Work out the finished part from the listing and answer in its coordinate system (mm). A direction names the side the tool comes from. Coordinates: 2 decimals unless noted, no trailing zeros. Write each loop counter-clockwise with the first axis right and the second up, starting at its lowest first coordinate (ties: lowest second). Pieces come first, ordered by that corner, then holes. Notation, with made-up numbers: (86.25, 8) - (110.25, 8) arc R26 ccw to (110.25, 42) - close; hole circle Ø7 at (44, 26). An arc over 180 degrees is marked (long way). Use one line per item in the form item = value. Start each with the question number.
Item 1: A cutting plane is placed at B-B (y = 130.5). Write down the section's boundary in (x, z), then the cut area to 3 significant figures.
Item 2: A cutting plane is placed at A-A (z = -21.5). Write down the section's boundary in (x, y), then the cut area to 3 significant figures.
Item 3: Given pin 1 (7 mm diameter, centred on x = 115, z = -28, fed in from -Y); pin 2 (7 mm diameter, centred on x = 113.5, z = -38.5, fed in from +Y); pin 3 (1.5 mm diameter, centred on x = 97.5, y = 41.5, fed in from -Z), each flat-ended and moving along its own axis, determine where each tip first touches the part or whether it passes through.
Item 4: Determine the mould class of faces 5 (the flat face through (70, 140, -9)), 6 (the flat face through (14, 75, -40)), 7 (the flat face through (123, 25, -8)) for opening direction X: released by +X, released by -X, zero draft, split by the parting line, or undercut.
Item 5: Consider probe 1 along X at (y, z) = (61.5, -22); probe 2 along Y at (x, z) = (16.5, -53.5); probe 3 along X at (y, z) = (71, -56). Determine where each line is inside the solid, lowest interval first.
Item 6: For faces 1 (the flat face through (19, 70, -41)), 2 (the flat face through (10, 108, -40)), 3 (the flat face through (120, 32, -41)), 4 (the flat face through (126, 50, -4)), determine the directions among +Z, -Z, +X, -X, +Y, -Y from which every point of the face is accessible in a straight line to the end or side of a thin tool.
Item 7: A cutting plane is placed at C-C (x = 71). Write down the section's boundary in (y, z).
Item 8: A cutting plane is placed at D-D (y = 24.5). Write down the section's boundary in (x, z).
from build123d import *

# Parameters (mm, degrees)
SKETCH1_W           = 130
SKETCH1_H           = 90
BOSS_EXTRUDE1_DEPTH = 140
SKETCH3_W           = 110
SKETCH3_H           = 70
CUT_EXTRUDE1_DEPTH  = 212.187120819
SKETCH4_W           = 110
SKETCH4_H           = 70
SKETCH4_W_2         = 92
SKETCH4_H_2         = 52
BOSS_EXTRUDE2_DEPTH = 75
SKETCH5_W           = 110
SKETCH5_H           = 70
SKETCH5_W_2         = 92
SKETCH5_H_2         = 52
CUT_EXTRUDE2_DEPTH  = 65
SKETCH6_W           = 130
SKETCH6_H           = 140
CUT_EXTRUDE3_DEPTH  = 19
SKETCH7_W           = 92
SKETCH7_H           = 10
CUT_EXTRUDE4_DEPTH  = 9
CUT_EXTRUDE5_DEPTH  = 50


with BuildPart() as part:
    # Sketch1 → Boss-Extrude1 (new body)
    with BuildSketch(Plane(origin=(0, 0, 0), x_dir=(1, 0, 0), z_dir=(0, 1, 0))):
        with Locations((65, 45)):
            Rectangle(SKETCH1_W, SKETCH1_H)
    extrude(amount=BOSS_EXTRUDE1_DEPTH)

    # Sketch3 → Cut-Extrude1 (cut, through all)
    with BuildSketch(Plane(origin=(0, 140, 0), x_dir=(1, 0, 0), z_dir=(0, 1, 0))):
        with Locations((65, 45)):
            Rectangle(SKETCH3_W, SKETCH3_H)
    extrude(amount=-CUT_EXTRUDE1_DEPTH, mode=Mode.SUBTRACT)

    # Sketch4 → Boss-Extrude2 (add)
    with BuildSketch(Plane.XZ):
        with Locations((65, -45)):
            Rectangle(SKETCH4_W, SKETCH4_H)
        with Locations((65, -45)):
            Rectangle(SKETCH4_W_2, SKETCH4_H_2, mode=Mode.SUBTRACT)
    extrude(amount=-BOSS_EXTRUDE2_DEPTH)

    # Sketch5 → Cut-Extrude2 (cut)
    with BuildSketch(Plane.XZ):
        with Locations((65, -45)):
            Rectangle(SKETCH5_W, SKETCH5_H)
        with Locations((65, -45)):
            Rectangle(SKETCH5_W_2, SKETCH5_H_2, mode=Mode.SUBTRACT)
    extrude(amount=-CUT_EXTRUDE2_DEPTH, mode=Mode.SUBTRACT)

    # Sketch6 → Cut-Extrude3 (cut)
    with BuildSketch(Plane(origin=(0, 0, -90), x_dir=(-1, 0, 0), z_dir=(0, 0, -1))):
        with Locations((-65, 70)):
            Rectangle(SKETCH6_W, SKETCH6_H)
    extrude(amount=-CUT_EXTRUDE3_DEPTH, mode=Mode.SUBTRACT)

    # Sketch7 → Cut-Extrude4 (cut)
    with BuildSketch(Plane(origin=(0, 0, -19), x_dir=(-1, 0, 0), z_dir=(0, 0, -1))):
        with Locations((-65, 70)):
            Rectangle(SKETCH7_W, SKETCH7_H)
    extrude(amount=-CUT_EXTRUDE4_DEPTH, mode=Mode.SUBTRACT)

    # Sketch8 → Cut-Extrude5 (cut)
    with BuildSketch(Plane(origin=(0, 0, 0), x_dir=(1, 0, 0), z_dir=(0, 1, 0))):
        Polygon((130, 0), (130, 15), (115, 0), align=None)
    extrude(amount=CUT_EXTRUDE5_DEPTH, mode=Mode.SUBTRACT)


solid = part.part
Answer:
q1.outline = (0, -71) - (10, -71) - (10, -10) - (120, -10) - (120, -71) - (130, -71) - (130, 0) - (0, 0) - close
q1.area = 2,520 mm²
q2.outline = (0, 0) - (10, 0) - (10, 65) - (19, 65) - (19, 75) - (10, 75) - (10, 140) - (0, 140) - close; (111, 65) - (120, 65) - (120, 0) - (130, 0) - (130, 140) - (120, 140) - (120, 75) - (111, 75) - close
q2.area = 2,980 mm²
q3.pin_1 = 65
q3.pin_2 = 75
q3.pin_3 = -10
q4.face_5 = zero draft
q4.face_6 = undercut
q4.face_7 = released by +X
q5.probe_1 = 0 to 10, 120 to 130
q5.probe_2 = 65 to 75
q5.probe_3 = 0 to 19, 111 to 130
q6.face_1 = -Z, +Y, -Y
q6.face_2 = -Z, +Y
q6.face_3 = -Z, -Y
q6.face_4 = +Z, +X, -Y
q7.outline = (0, -10) - (140, -10) - (140, 0) - (0, 0) - close
q8.outline = (0, -71) - (10, -71) - (10, -10) - (120, -10) - (120, -71) - (130, -71) - (130, -15) - (115, 0) - (0, 0) - close
